Geometry: final body of the model. Coordinates: model frame, mm. A direction names the side the tool comes from. Coordinates: 2 decimals unless noted, no trailing zeros. Order: outer loops, then holes, each group sorted by start corner. A loop starts at its lowest first (then second) coordinate and runs counter-clockwise, first axis right, second up. Notation, with made-up numbers: (6.5, 49.5) -> (17.5, 49.5) arc R16 ccw to (17.5, 79.5) -> close; hole circle Ø11 at (25, 10). An arc over 180 degrees is marked (long way). Answer in a Markdown table with one row per item. Add a question column.
1) Ray query, line 1 (X direction, y = 3.5, z = 10); line 2 (Z direction, x = 2.75, y = -1.75); line 3 (Z direction, x = -13.25, y = 2.5). Return the intervals inside material, ascending. Write a range as from..to.
2) Pull-direction query (Z, two-part tool) for faces 4 (the face through (0, 0, 0)), 5 (the face through (0, -2, 43.867)), 6 (the face through (0, 2, -15)); classes: +Z half, -Z half, draft (parallel to the pull), parting line (faces both ways), or undercut.
3) Set-up query: faces 1 (the face through (-10, 3, 0)), 2 (the face through (9, 3, 0)), 3 (the face through (0, 3, 29)). Return all of +Z, -Z, +X, -X, +Y, -Y with unobstructed straight access to the full face (end or side cutting, diameter ignored); none if empty.
4) Section query D-D on x = -8.5. Return the cut outline in (y, z), then the cut area to 3 significant figures.
5) Section query A-A on z = -6.5. Return the cut outline in (x, y), then the cut area to 3 significant figures.
6) Contact query for flat-ended pins moving along their axis: P1, Ø12.5, axis at x = 9, z = 2, coming from the +Y side; P2, Ø9, axis at x = 1, z = 30.5, coming from the -Y side; P3, Ø5, axis at x = -9.5, z = -5, coming from the +Y side; P4, Ø1.5, axis at x = 4.5, y = 2, coming from the +Z side. Output: stop coordinate, or through.
7) Section query B-B on x = 0.25. Return the cut outline in (y, z).
8) Section query C-C on y = -1.5. Return the cut outline in (x, z).
```python
from build123d import *

# Parameters (mm, degrees)
CROQUIS1_W              = 30
CROQUIS1_H              = 30
SALIENTE_EXTRUIR1_DEPTH = 3
CROQUIS2_W              = 8.214533593
CROQUIS2_H              = 58.866686573
SALIENTE_EXTRUIR2_DEPTH = 3
CROQUIS3_W              = 8.214533593
CROQUIS3_H              = 13.391786962
SALIENTE_EXTRUIR3_DEPTH = 3


with BuildPart() as part:
    # Croquis1 → Saliente-Extruir1 (new body)
    with BuildSketch(Plane(origin=(0, 0, 0), x_dir=(1, 0, 0), z_dir=(0, 1, 0))):
        Rectangle(CROQUIS1_W, CROQUIS1_H)
    extrude(amount=SALIENTE_EXTRUIR1_DEPTH)

    # Croquis2 → Saliente-Extruir2 (add)
    with BuildSketch(Plane(origin=(0, 3, 0), x_dir=(1, 0, 0), z_dir=(0, 1, 0))):
        with Locations((-0.441980957, -14.433343287)):
            Rectangle(CROQUIS2_W, CROQUIS2_H)
    extrude(amount=SALIENTE_EXTRUIR2_DEPTH)

    # Croquis3 → Saliente-Extruir3 (add)
    with BuildSketch(Plane.XY.offset(43.866686573)):
        with Locations((-0.441980957, -0.695893481)):
            Rectangle(CROQUIS3_W, CROQUIS3_H)
    extrude(amount=SALIENTE_EXTRUIR3_DEPTH)


solid = part.part
```
Result:
| question | item | result |
|---|---|---|
| 1 | line 1 | -4.55..3.67 |
| 1 | line 2 | 43.87..46.87 |
| 1 | line 3 | -15..15 |
| 2 | face 4 | draft |
| 2 | face 5 | undercut |
| 2 | face 6 | -Z half |
| 3 | face 1 | +Z, -Z, -X, +Y |
| 3 | face 2 | +Z, -Z, +X, +Y |
| 3 | face 3 | +X, -X, -Y |
| 4 | outline | (0, -15) -> (3, -15) -> (3, 15) -> (0, 15) -> close |
| 4 | area | 90.0 mm2 |
| 5 | outline | (-15, 0) -> (15, 0) -> (15, 3) -> (3.67, 3) -> (3.67, 6) -> (-4.55, 6) -> (-4.55, 3) -> (-15, 3) -> close |
| 5 | area | 115 mm2 |
| 6 | P1 | y = 6 |
| 6 | P2 | y = 3 |
| 6 | P3 | y = 3 |
| 6 | P4 | z = 15 |
| 7 | outline | (-7.39, 43.87) -> (3, 43.87) -> (3, 15) -> (0, 15) -> (0, -15) -> (6, -15) -> (6, 46.87) -> (-7.39, 46.87) -> close |
| 8 | outline | (-4.55, 43.87) -> (3.67, 43.87) -> (3.67, 46.87) -> (-4.55, 46.87) -> close |
